```python
from build123d import *

# Parameters (mm, degrees)
SKETCH2_W           = 112.649
SKETCH2_H           = 104.648
SKETCH2_R           = 3.81
SKETCH2_W_2         = 74.389
SKETCH2_H_2         = 69.53
BOSS_EXTRUDE5_DEPTH = 12.7
SKETCH2_4_W         = 74.389
SKETCH2_4_H         = 10
SKETCH2_4_R         = 2.5
BOSS_EXTRUDE7_DEPTH = 8.89


with BuildPart() as part:
    # Sketch2 → Boss-Extrude5 (new body)
    with BuildSketch(Plane(origin=(0, 0, 0), x_dir=(1, 0, 0), z_dir=(0, 1, 0))):
        with Locations((56.3245, 52.324)):
            Rectangle(SKETCH2_W, SKETCH2_H)
        with Locations((12.065, 96.52)):
            Circle(SKETCH2_R, mode=Mode.SUBTRACT)
        with Locations((12.065, 58.928)):
            Circle(SKETCH2_R, mode=Mode.SUBTRACT)
        with Locations((12.065, 45.72)):
            Circle(SKETCH2_R, mode=Mode.SUBTRACT)
        with Locations((12.065, 8.128)):
            Circle(SKETCH2_R, mode=Mode.SUBTRACT)
        with Locations((100.584, 8.128)):
            Circle(SKETCH2_R, mode=Mode.SUBTRACT)
        with Locations((100.584, 45.72)):
            Circle(SKETCH2_R, mode=Mode.SUBTRACT)
        with Locations((100.584, 58.928)):
            Circle(SKETCH2_R, mode=Mode.SUBTRACT)
        with Locations((100.584, 96.52)):
            Circle(SKETCH2_R, mode=Mode.SUBTRACT)
        with Locations((56.3245, 52.324)):
            Rectangle(SKETCH2_W_2, SKETCH2_H_2, mode=Mode.SUBTRACT)
    extrude(amount=BOSS_EXTRUDE5_DEPTH)

    # Sketch2_4 → Boss-Extrude7 (add)
    with BuildSketch(Plane(origin=(0, 0, 0), x_dir=(1, 0, 0), z_dir=(0, 1, 0))):
        with Locations((56.3245, 82.089)):
            Rectangle(SKETCH2_4_W, SKETCH2_4_H)
        with Locations((31.533666667, 82.089)):
            Circle(SKETCH2_4_R, mode=Mode.SUBTRACT)
        with Locations((56.341, 82.089)):
            Circle(SKETCH2_4_R, mode=Mode.SUBTRACT)
        with Locations((81.148333333, 82.089)):
            Circle(SKETCH2_4_R, mode=Mode.SUBTRACT)
        with Locations((56.3245, 22.559)):
            Rectangle(SKETCH2_4_W, SKETCH2_4_H)
        with Locations((31.533666667, 22.559)):
            Circle(SKETCH2_4_R, mode=Mode.SUBTRACT)
        with Locations((56.341, 22.559)):
            Circle(SKETCH2_4_R, mode=Mode.SUBTRACT)
        with Locations((81.148333333, 22.559)):
            Circle(SKETCH2_4_R, mode=Mode.SUBTRACT)
    extrude(amount=BOSS_EXTRUDE7_DEPTH)


solid = part.part
```
The model under review builds one solid part; all positions refer to its coordinate system, in mm. A direction names the side the tool comes from. Give positions to 0.01 mm unless a question says otherwise; leave off trailing zeros. Write each loop counter-clockwise with the first axis right and the second up, starting at its lowest first coordinate (ties: lowest second). Pieces come first, ordered by that corner, then holes. Notation, with made-up numbers: (44.25, -35) - (79.25, -35) arc R15 ccw to (79.25, -14) - close; hole circle Ø10 at (-17, 54.25). An arc over 180 degrees is marked (long way). Answer in a Markdown table with one row per item. Add a question column.
1. Tool access review of faces 1 (the flat face through (0, 6, -52)), 2 (the flat face through (56, 11, -17.559)): name each direction out of +Z, -Z, +X, -X, +Y, -Y from which nothing blocks a thin tool from reaching the whole face with its end or side.
2. We need section D-D on y = 10.5. State how many separate pieces and enclosed holes the cut face has, then the cut area to 3 significant figures.
3. Draft analysis for pull direction Z (two halves, no side actions). For faces 3 (the flat face through (56, 8.89, -26)), 4 (the cylindrical face through (104.22, 6.26, -9.27)), 5 (the flat face through (112.649, 6, -52)), 6 (the flat face through (56, 6, -104.648)), state which applies: +Z half, -Z half, draft (parallel to the pull), parting line (faces both ways), or undercut.
4. We need section C-C on z = -45.72. Write out the cut boundary in (x, y) (3 decimals), then the cut area to 3 significant figures.
5. Wall thickness on line 1 along X through (y, z) = (5, -8.5); line 2 along X through (y, z) = (6.75, -45.72) (3 decimals); line 3 along Z through (x, y) = (20, 10.75): over which ranges is each line inside the solid? List them lowest first. Write a range as [from, to].
6. We need section B-B on x = 64.5. Write out the cut boundary in (y, z).
7. Insertion check: P1, Ø6, axis at x = 56.341, z = -82.089, coming from the -Y side; P2, Ø3, axis at x = 38.5, z = -74.5, coming from the -Y side; P3, Ø5, axis at x = 63, z = -22, coming from the +Y side. Each pin has a flat end and moves straight along its axis. Give the tip position at first contact, or say it passes through.
8. We need section A-A on z = -96.52. Write out the cut boundary in (x, y) (3 decimals).
Ans:
| question | item | result |
|---|---|---|
| 1 | face 1 | +Z, -Z, -X, +Y, -Y |
| 1 | face 2 | +Y |
| 2 | separate pieces | 1 |
| 2 | enclosed holes | 9 |
| 2 | area | 6,250 mm^2 |
| 3 | face 3 | undercut |
| 3 | face 4 | undercut |
| 3 | face 5 | draft |
| 3 | face 6 | -Z half |
| 4 | outline | (0, 0) - (8.255, 0) - (8.255, 12.7) - (0, 12.7) - close; (15.875, 0) - (19.13, 0) - (19.13, 12.7) - (15.875, 12.7) - close; (93.519, 0) - (96.774, 0) - (96.774, 12.7) - (93.519, 12.7) - close; (104.394, 0) - (112.649, 0) - (112.649, 12.7) - (104.394, 12.7) - close |
| 4 | area | 292 mm^2 |
| 5 | line 1 | x = [0, 8.27], [15.86, 96.79], [104.38, 112.65] |
| 5 | line 2 | x = [0, 8.255], [15.875, 19.13], [93.519, 96.774], [104.394, 112.649] |
| 5 | line 3 | z = [-104.65, -87.09], [-17.56, 0] |
| 6 | outline | (0, -104.65) - (12.7, -104.65) - (12.7, -87.09) - (8.89, -87.09) - (8.89, -77.09) - (0, -77.09) - close; (0, -27.56) - (8.89, -27.56) - (8.89, -17.56) - (12.7, -17.56) - (12.7, 0) - (0, 0) - close |
| 7 | P1 | stops at y = 0 |
| 7 | P2 | passes through |
| 7 | P3 | stops at y = 8.89 |
| 8 | outline | (0, 0) - (8.255, 0) - (8.255, 12.7) - (0, 12.7) - close; (15.875, 0) - (96.774, 0) - (96.774, 12.7) - (15.875, 12.7) - close; (104.394, 0) - (112.649, 0) - (112.649, 12.7) - (104.394, 12.7) - close |
